Design review of the part built by this model. Coordinates are the model's own, in mm. A direction names the side the tool comes from. Give positions to 0.01 mm unless a question says otherwise; leave off trailing zeros. Write each loop counter-clockwise with the first axis right and the second up, starting at its lowest first coordinate (ties: lowest second). Pieces come first, ordered by that corner, then holes. Notation, with made-up numbers: (-0.5, 32.5) - (56.5, 32.5) arc R19 cw to (56.5, 55.5) - close; hole circle Ø11 at (29.5, 22.5). An arc over 180 degrees is marked (long way). Write each question's results on one line, items separated by ' | '. Start each with the question number.
from build123d import *

# Parameters (mm, degrees)
EXTRUDE_1_DEPTH     = 11
SKETCH_2_R          = 10
CUT_EXTRUDE_1_DEPTH = 11
FILLET_1_R          = 2
CUT_EXTRUDE_2_DEPTH = 20
SKETCH_6_R          = 2
CUT_EXTRUDE_4_DEPTH = 33


with BuildPart() as part:
    # 草图1 → 凸台-拉伸1 (new body)
    with BuildSketch(Plane.XY):
        with BuildLine():
            Line((-44.744635323, -4.787234043), (-19.886504588, -237.127659574))
            ThreePointArc((-19.886504588, -237.127659574), (0, -255), (19.886504588, -237.127659574))
            Line((19.886504588, -237.127659574), (44.744635323, -4.787234043))
            ThreePointArc((44.744635323, -4.787234043), (0, 45), (-44.744635323, -4.787234043))
        make_face()
    extrude(amount=EXTRUDE_1_DEPTH)

    # 草图2 → 切除-拉伸1 (cut)
    with BuildSketch(Plane(origin=(0, 0, 0), x_dir=(-1, 0, 0), z_dir=(0, 0, -1))):
        with Locations((0, -235.836034695)):
            Circle(SKETCH_2_R)
    extrude(amount=-CUT_EXTRUDE_1_DEPTH, mode=Mode.SUBTRACT)

    # 圆角1
    fillet_1_edges = [part.edges().sort_by_distance(p)[0] for p in [
        (0, -255, 11),
        (32.315569956, -120.957446809, 11),
        (0, 45, 11),
        (32.315569956, -120.957446809, 0),
        (0, -255, 0),
        (-32.315569956, -120.957446809, 0),
        (0, 45, 0),
        (-32.315569956, -120.957446809, 11),
    ]]
    fillet(fillet_1_edges, radius=FILLET_1_R)

    # 草图4 → 切除-拉伸2 (cut)
    with BuildSketch(Plane(origin=(0, 0, 0), x_dir=(-1, 0, 0), z_dir=(0, 0, -1))):
        with BuildLine():
            Line((-21.759824224, -44.682312886), (-3.625991278, -214.173032358))
            ThreePointArc((-3.625991278, -214.173032358), (0.015295132, -212.723088949), (3.615338262, -214.272602446))
            Line((3.615338262, -214.272602446), (21.759824224, -44.682312886))
            ThreePointArc((21.759824224, -44.682312886), (0, -50.060383894), (-21.759824224, -44.682312886))
        make_face()
    extrude(amount=-CUT_EXTRUDE_2_DEPTH, mode=Mode.SUBTRACT)

    # 草图6 → 切除-拉伸4 (cut)
    with BuildSketch(Plane.XY.offset(11)):
        with Locations((-16.789244382, 3.960274368)):
            Circle(SKETCH_6_R)
        with Locations((-4.964923982, 16.52004933)):
            Circle(SKETCH_6_R)
        with Locations((11.8243204, 12.559774961)):
            Circle(SKETCH_6_R)
        with Locations((16.789244382, -3.960274368)):
            Circle(SKETCH_6_R)
        with Locations((4.964923982, -16.52004933)):
            Circle(SKETCH_6_R)
        with Locations((-11.8243204, -12.559774961)):
            Circle(SKETCH_6_R)
    extrude(amount=-CUT_EXTRUDE_4_DEPTH, mode=Mode.SUBTRACT)


solid = part.part
Q1. Machinability: for faces 5 (the face through (-12.56, -130.66, 5.42)), 6 (the face through (-31.574, -122.523, 10.399)), which of the approach directions +Z, -Z, +X, -X, +Y, -Y give a long, thin tool a straight path to every point of the face, cutting with its end or side? Answer none if there is none.
Q2. Insertion check: P1, Ø4, axis at y = -85.5, z = 6, coming from the -X side; P2, Ø2, axis at y = 0.5, z = 4.5, coming from the +X side; P3, Ø6, axis at x = 4, z = 6.5, coming from the -Y side (3 decimals). Each pin has a flat end and moves straight along its axis. Give the tip position at first contact, or say it passes through.
Q3. Add section B-B on z = 6.5. Count the separate pieces of the cut face and the enclosed holes in it, plus the area to 3 significant figures.
Q4. For line 1 along X through (y, z) = (-186, 3.25); line 2 along X through (y, z) = (-201.5, 1.25); line 3 along X through (y, z) = (-28.5, 4.25), list the stretches that pass through material, from the lowest coordinate up. Write a range as [from, to].
Q5. Add section A-A on x = 0. State the section outline as (y, z) points, plus the area to 3 significant figures.
Q6. The part is to be moulded in two halves that separate along Y. For faces 1 (the face through (-31.544, -122.52, 0.57)), 2 (the face through (0.041, -212.723, 5.423)), 3 (the face through (12.82, -128.24, 5.42)), 4 (the face through (-20, -70, 11)), say which applies: +Y half, -Y half, draft (parallel to the pull), parting line (faces both ways), or undercut.
Result:
1) face 5: +Z, -Z | face 6: +Z, -X, -Y
2) P1: stops at x = -36.32 | P2: stops at x = 45 | P3: stops at y = -254.975
3) separate pieces: 1 | enclosed holes: 8 | area: 14,600 mm²
4) line 1: x = [-25.36, -6.64], [6.64, 25.36] | line 2: x = [-23.55, -4.98], [4.98, 23.55] | line 3: x = [-42.21, 42.21]
5) outline: (-255, 2) arc R2 ccw to (-253, 0) - (-245.84, 0) - (-245.84, 11) - (-253, 11) arc R2 ccw to (-255, 9) - close; (-225.84, 0) - (-212.72, 0) - (-212.72, 11) - (-225.84, 11) - close; (-50.06, 0) - (43, 0) arc R2 ccw to (45, 2) - (45, 9) arc R2 ccw to (43, 11) - (-50.06, 11) - close | area: 1,290 mm²
6) face 1: -Y half | face 2: undercut | face 3: undercut | face 4: draft
